Can you work these out from the model? Positions are in its coordinate system, mm. Give positions to 0.01 mm unless a question says otherwise; leave off trailing zeros. Write each loop counter-clockwise with the first axis right and the second up, starting at its lowest first coordinate (ties: lowest second). Pieces come first, ordered by that corner, then holes.
Autodesk Inventor part; units mm, degrees
ref_plane "YZ Plane" through (0, 0, 0) normal (1, 0, 0) x (0, 1, 0)
ref_plane "XZ Plane" through (0, 0, 0) normal (0, 1, 0) x (-1, 0, 0)
ref_plane "XY Plane" through (0, 0, 0) normal (0, 0, 1) x (1, 0, 0)
sketch "Sketch1" plane through (0, 0, 0) normal (0, 0, 1) x (1, 0, 0)
  line L0 (-125, -110) -> (-125, 110)
  line L1 (-125, 110) -> (125, 110)
  line L2 (125, 110) -> (125, -110)
  line L3 (125, -110) -> (-125, -110)
  line L4 (-125, -110) -> (125, 110) construction
  line L5 (-125, 110) -> (125, -110) construction
  point P0 (0, 0)
  dimension "d0" = 220
  dimension "d1" = 250
extrude "Extrusion1" add sketch "Sketch1" along normal blind 10
sketch "Sketch2" plane through (0, 0, 0) normal (0, 0, -1) x (-1, 0, 0)
  line L0 (50, 100) -> (-50, 100)
  line L1 (-50, 100) -> (-50, -100)
  line L2 (-50, -100) -> (50, -100)
  line L3 (50, -100) -> (50, 100)
  line L4 (50, 100) -> (-50, -100) construction
  line L5 (-50, 100) -> (50, -100) construction
  line L6 (-125, -110) -> (-125, 110)
  line L7 (125, -110) -> (-125, -110)
  point P0 (0, 0)
  point P1 (50, -50)
  point P2 (50, 70)
  point P3 (-50, -50)
  point P4 (-50, 70)
  dimension "d4" = 75
  dimension "d5" = 10
  dimension "d6" = 50
  dimension "d7" = 30
hole "Hole1" at (-50, -50, 0) at (-50, 70, 0) at (50, -50, 0) at (50, 70, 0) at (50, -100, 0) at (-50, -100, 0) direction (0, 0, 1) diameter 4.5 end through all
sketch "Sketch3" plane through (0, 0, 10) normal (0, 0, 1) x (1, 0, 0)
  line L0 (109.42, -76) -> (119.92, -76)
  line L1 (109.42, -76) -> (109.42, -90)
  line L2 (109.42, -90) -> (119.92, -90)
  line L3 (119.92, -90) -> (119.92, -76)
  circle A0 centre (115.92, -83) radius 3
  line L4 (79.92, -90) -> (90.42, -90)
  line L5 (90.42, -90) -> (90.42, -76)
  line L6 (79.92, -76) -> (90.42, -76)
  line L7 (79.92, -76) -> (79.92, -90)
  circle A1 centre (83.92, -83) radius 3
  line L8 (34, -69) -> (34, -93)
  line L9 (18, -69) -> (34, -69)
  line L10 (18, -93) -> (18, -69)
  line L11 (34, -93) -> (18, -93)
  circle A2 centre (26.5, -81) radius 5
  circle A3 centre (-26.5, -81) radius 5
  line L12 (-34, -93) -> (-34, -69)
  line L13 (-18, -93) -> (-34, -93)
  line L14 (-18, -93) -> (-18, -69)
  line L15 (-34, -69) -> (-18, -69)
  circle A4 centre (-26.5, -81) radius 5
  line L16 (-79.92, -76) -> (-90.42, -76)
  line L17 (-90.42, -76) -> (-90.42, -90)
  line L18 (-79.92, -90) -> (-90.42, -90)
  line L19 (-79.92, -90) -> (-79.92, -76)
  circle A5 centre (-83.92, -83) radius 3
  line L20 (-109.42, -90) -> (-119.92, -90)
  line L21 (-109.42, -90) -> (-109.42, -76)
  line L22 (-109.42, -76) -> (-119.92, -76)
  line L23 (-119.92, -76) -> (-119.92, -90)
  circle A6 centre (-115.92, -83) radius 3
  line L24 (-34, 70) -> (-34, 90)
  line L25 (-18, 70) -> (-34, 70)
  line L26 (-18, 90) -> (-18, 70)
  line L27 (-34, 90) -> (-18, 90)
  circle A7 centre (-26.5, 80) radius 4.5
  line L28 (34, 90) -> (34, 70)
  line L29 (18, 90) -> (34, 90)
  line L30 (18, 90) -> (18, 70)
  line L31 (34, 70) -> (18, 70)
  circle A8 centre (26.5, 80) radius 4.5
  point P0 (0, 0)
extrude "Extrusion2" cut sketch "Sketch3" against normal blind 10 contours A0 | A1 | A2 | A3 | A5 | A6 | A7 | A8
sketch "Sketch4" plane through (0, 0, 0) normal (0, 0, -1) x (-1, 0, 0)
  circle A0 centre (-83.92, -83) radius 3
  circle A1 centre (115.92, -83) radius 3
  circle A2 centre (26.5, 80) radius 4.5
  circle A3 centre (-26.5, -81) radius 5
  circle A4 centre (-115.92, -83) radius 3
  circle A5 centre (83.92, -83) radius 3
  circle A6 centre (-26.5, 80) radius 4.5
  circle A7 centre (26.5, -81) radius 5
  circle A8 centre (-50, -100) radius 2.25
  circle A9 centre (-50, -50) radius 2.25
  circle A10 centre (50, -50) radius 2.25
  circle A11 centre (50, 70) radius 2.25
  circle A12 centre (-50, 70) radius 2.25
  circle A13 centre (50, -100) radius 2.25
  line L0 (-125, -110) -> (-125, 110)
  line L1 (125, -110) -> (-125, -110)
  line L2 (125, 110) -> (125, -110)
  line L3 (-125, 110) -> (125, 110)
  line L4 (-175, 60) -> (-75, 60)
  line L5 (-75, 60) -> (-75, -60)
  line L6 (-75, -60) -> (-175, -60)
  line L7 (-175, -60) -> (-175, 60)
  line L8 (-125, -110) -> (-125, 110)
  line L9 (-175, 60) -> (-75, -60) construction
  line L10 (-75, 60) -> (-175, -60) construction
  point P0 (0, 0)
  point P1 (-125, 0)
  point P2 (-125, 60)
  point P3 (-125, -60)
  dimension "d17" = 100
  dimension "d18" = 120
extrude "Extrusion3" cut sketch "Sketch4" against normal blind 67.5 contours L0 L4 L5 L6
mirror "Mirror1" about plane through (0, 0, 0) normal (1, 0, 0) of "Extrusion3"
fillet "Fillet1" radius 15.25 4 edges at (75, -60, 5) (75, 60, 5) (-75, -60, 5) (-75, 60, 5)
chamfer "Chamfer1" distance 12 angle 45 4 edges at (125, -60, 5) (125, 60, 5) (-125, 60, 5) (-125, -60, 5)
properties part number "08_Tam_truc_Z" material "Stainless Steel, Austenitic"
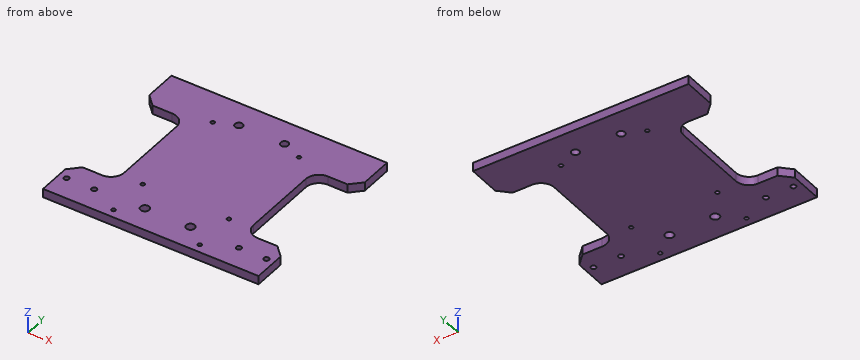
1) Suppose I cut it at D-D on y = 29. Write out the boundary of the cut face in (x, z), plus the area to 3 significant figures.
Values follow:
outline: (-75, 0) - (75, 0) - (75, 10) - (-75, 10) - close
area: 1,500 mm2
2) Suppose I cut it at B-B on y = 80. Write out the boundary of the cut face in (x, z), plus the area to 3 significant figures.
Values follow:
outline: (-125, 0) - (-31, 0) - (-31, 10) - (-125, 10) - close; (-22, 0) - (22, 0) - (22, 10) - (-22, 10) - close; (31, 0) - (125, 0) - (125, 10) - (31, 10) - close
area: 2,320 mm2
3) Please list where these lines run through material, in increasing order: L1, parallel to Y at x = 50, z = 7; L2, parallel to Y at x = -26.5, z = 6.5; L3, parallel to Y at x = -115.92, z = 7.5.
Values follow:
L1: y = -110 to -102.25, -97.75 to -52.25, -47.75 to 67.75, 72.25 to 110
L2: y = -110 to -86, -76 to 75.5, 84.5 to 110
L3: y = -110 to -86, -80 to -62.92, 62.92 to 110
4) Suppose I cut it at A-A on x = 26.5. Write out the boundary of the cut face in (y, z).
Values follow:
outline: (-110, 0) - (-86, 0) - (-86, 10) - (-110, 10) - close; (-76, 0) - (75.5, 0) - (75.5, 10) - (-76, 10) - close; (84.5, 0) - (110, 0) - (110, 10) - (84.5, 10) - close
5) For pin 1 Ø7 at (x, y) = (-83.92, -83) entering from +Z; pin 2 Ø5 at (y, z) = (8.5, 2.5) entering from +X; pin 3 Ø4 at (y, z) = (-58.5, 8.5) entering from -X, each with a flat end and sliding along its axis, tell me the tip position at first contact or that it passes through.
Values follow:
pin 1: stops at z = 10
pin 2: stops at x = 75
pin 3: stops at x = -113.5
6) Suppose I cut it at C-C on z = 7.5. State how many separate pieces and enclosed holes the cut face has, plus the area to 3 significant figures.
Values follow:
separate pieces: 1
enclosed holes: 14
area: 42,400 mm2
